Work out the finished part from the listing and answer in its coordinate system (mm). Face numbers are marked on the shaded views. Coordinates: 2 decimals unless noted, no trailing zeros. Loops run counter-clockwise (first coordinate to the right, second up) from the corner with the lowest first, then second, coordinate; pieces in that order, holes last. Notation, with made-up numbers: (9.25, -34) -> (53.25, -34) arc R22 cw to (53.25, -18) -> close; hole circle Ø8 at (1, 14). An arc over 180 degrees is marked (long way). Use a Markdown table: item, result. Add a question column.
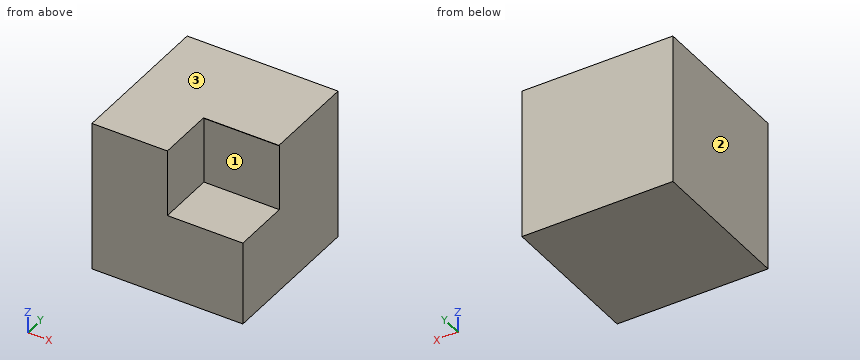
```python
from build123d import *

# Parameters (mm, degrees)
F0_W     = 50.793938
F0_H     = 50.793935
F1_DEPTH = 50.8
F3_DEPTH = 25.4


with BuildPart() as f1:
    # F0 (on Front) → F1 (new body)
    with BuildSketch(Plane.XZ):
        with Locations((-25.396969, 25.396967)):
            Rectangle(F0_W, F0_H)
    extrude(amount=F1_DEPTH)

    # F2 (on Right) → F3 (cut)
    with BuildSketch(Plane.YZ):
        Polygon((-31.325877, 50.512649), (-52.65988, 79.119146), (-72.913677, 79.119146), (-72.913677, 55.439733), (-51.039577, 28.238516), (-31.325877, 28.238516), align=None)
    extrude(amount=-F3_DEPTH, mode=Mode.SUBTRACT)


solid = f1.part
```
Item 1: Find the intervals of material crossed by probe 1 along Y at (x, z) = (-3.5, 46); probe 2 along Z at (x, y) = (-5.5, -43); probe 3 along X at (y, z) = (-36.5, 43), in increasing order.
Item 2: Section C-C (y = -46.5) is taken. Determine the outline of the cut face in (x, z).
Item 3: Section A-A (z = 32) is taken. Determine the outline of the cut face in (x, y).
Item 4: Section B-B (x = -24) is taken. Determine the outline of the cut face in (y, z).
Item 5: Given pin 1 (21.5 mm diameter, centred on y = -45.5, z = 42.5, fed in from +X); pin 2 (11 mm diameter, centred on x = -17, z = 36, fed in from -Y); pin 3 (21.5 mm diameter, centred on x = -10, y = -45, fed in from +Z), each flat-ended and moving along its own axis, determine where each tip first touches the part or whether it passes through.
Item 6: For a pull along Z with two mould halves and no side action, classify the marked faces 1, 2 and 3 as +Z half, -Z half, draft (parallel to the pull), parting line (faces both ways), or undercut.
Output:
| question | item | result |
|---|---|---|
| 1 | probe 1 | y = -31.33 to 0 |
| 1 | probe 2 | z = 0 to 28.24 |
| 1 | probe 3 | x = -50.79 to -25.4 |
| 2 | outline | (-50.79, 0) -> (0, 0) -> (0, 28.24) -> (-25.4, 28.24) -> (-25.4, 50.79) -> (-50.79, 50.79) -> close |
| 3 | outline | (-50.79, -50.8) -> (-25.4, -50.8) -> (-25.4, -31.33) -> (0, -31.33) -> (0, 0) -> (-50.79, 0) -> close |
| 4 | outline | (-50.8, 0) -> (0, 0) -> (0, 50.79) -> (-31.54, 50.79) -> (-31.33, 50.51) -> (-31.33, 28.24) -> (-50.8, 28.24) -> close |
| 5 | pin 1 | stops at x = -25.4 |
| 5 | pin 2 | stops at y = -31.33 |
| 5 | pin 3 | stops at z = 28.24 |
| 6 | face 1 | undercut |
| 6 | face 2 | draft |
| 6 | face 3 | +Z half |
